Check sheet for the modelled part. Datum: model origin and axes. Units: mm. A direction names the side the tool comes from. Coordinates: 2 decimals unless noted, no trailing zeros. Write each loop counter-clockwise with the first axis right and the second up, starting at its lowest first coordinate (ties: lowest second). Pieces come first, ordered by that corner, then holes. Notation, with made-up numbers: (51, 30) - (87, 30) arc R14 cw to (87, 35) - close; hole circle Ø6 at (6.5, -7). An arc over 180 degrees is marked (long way). Answer as CSV lines item,"result". Start each with the question number.
from build123d import *

# Parameters (mm, degrees)
SKETCH_1_R      = 4
SKETCH_1_R_2    = 2.5
EXTRUDE_1_DEPTH = 6


with BuildPart() as part:
    # 스케치1 → 보스-돌출1 (new body)
    # profile 1 of 4: a face of its own
    with BuildSketch(Plane.XY):
        with BuildLine():
            Line((4, -3.202328983), (4, 0))
            ThreePointArc((4, 0), (-3e-09, -4), (-4, 6e-09))
            Line((-4, 6e-09), (-4, -1.928017797))
            Line((-4, -1.928017797), (-11.877068301, -1.928017797))
            Line((-11.877068301, -1.928017797), (-11.877068301, -4.928017797))
            Line((-11.877068301, -4.928017797), (-6.12956889, -4.928017797))
            Line((-6.12956889, -4.928017797), (-6.12956889, -7.005884989))
            Line((-6.12956889, -7.005884989), (1.618982626, -7.005884989))
            Line((1.618982626, -7.005884989), (4, -3.202328983))
        make_face()
    # profile 2 of 4: a face of its own
    with BuildSketch(Plane.XY):
        Circle(SKETCH_1_R)
        Circle(SKETCH_1_R_2, mode=Mode.SUBTRACT)
    # profile 3 of 4: a face of its own
    with BuildSketch(Plane.XY):
        with BuildLine():
            Line((4, 15), (-0.018657753, 12.499853249))
            Line((-0.018657753, 12.499853249), (-0.018657753, 8.804925293))
            Line((-0.018657753, 8.804925293), (-4, 6.585919306))
            Line((-4, 6.585919306), (-4, 6e-09))
            ThreePointArc((-4, 6e-09), (3e-09, 4), (4, 0))
            Line((4, 0), (4, 15))
        make_face()
    # profile 4 of 4: a face of its own
    with BuildSketch(Plane.XY):
        with BuildLine():
            ThreePointArc((-6.12956889, -7.005884989), (-9.072577994, -15.066190234), (-6.302707776, -23.187621278))
            ThreePointArc((-6.302707776, -23.187621278), (-4.499421911, -23.894054073), (-2.999999998, -22.668239597))
            ThreePointArc((-2.999999998, -22.668239597), (-3.892893232, -13.892647551), (1.618982626, -7.005884989))
            Line((1.618982626, -7.005884989), (-6.12956889, -7.005884989))
        make_face()
    extrude(amount=EXTRUDE_1_DEPTH)


solid = part.part
(1) Release check for a two-part mould opening along Y. For faces 4 (the face through (-3.928, -14.014, 2.958)), 5 (the face through (-6.13, -6, 3)), 6 (the face through (-4.53, -23.9, 2.96)), 7 (the face through (-0.019, 11, 3)) record: pulls with the +Y half, pulls with the -Y half, needs draft (parallel to the pull), parting line crosses it, or undercut.
(2) Cross-section at D-D on y = 12. Record the boundary of the cut face in (x, z).
(3) Go/stop test with flat-tipped pins: P1, Ø1.7, axis at x = -9, z = 4, coming from the -Y side; P2, Ø3, axis at y = 2.5, z = 3.5, coming from the -X side; P3, Ø3, axis at x = 0, y = 0, coming from the -Z side; P4, Ø0.6, axis at y = -6, z = 4.5, coming from the -X side. Record where each tip stops, or that it passes through.
(4) Material ranges on probe 1 along X at (y, z) = (-2, 2.95); probe 2 along X at (y, z) = (3.5, 4.25); probe 3 along X at (y, z) = (10.5, 3.8), recorded low to high. Write a range as from..to.
(5) Cross-section at A-A on y = 0. Record the boundary of the cut face in (x, z).
(6) Cross-section at B-B on z = 3.6. Record the boundary of the cut face in (x, y), plus the area to 3 significant figures.
(7) Tool access check on faces 1 (the face through (-9, -4.928, 3)), 2 (the face through (-11.877, -3, 3)), 3 (the face through (-4, 2, 3)). Record the directions out of +Z, -Z, +X, -X, +Y, -Y that give a thin tool (end or side, any length) a straight path to the whole face; none if there is none.
(8) Cross-section at C-C on x = -3.5. Record the boundary of the cut face in (y, z), plus the area to 3 significant figures.
Checked values:
1,face 4,"undercut"
1,face 5,"undercut"
1,face 6,"pulls with the -Y half"
1,face 7,"needs draft"
2,outline,"(-0.02, 0) - (4, 0) - (4, 6) - (-0.02, 6) - close"
3,P1,"y = -19.99"
3,P2,"x = -4"
3,P3,"through"
3,P4,"x = -6.13"
4,probe 1,"-11.88..-1.5, 1.5..4"
4,probe 2,"-4..4"
4,probe 3,"-0.02..4"
5,outline,"(-4, 0) - (-2.5, 0) - (-2.5, 6) - (-4, 6) - close; (2.5, 0) - (4, 0) - (4, 6) - (2.5, 6) - close"
6,outline,"(-11.88, -4.93) - (-6.13, -4.93) - (-6.13, -7.01) arc R12.89 ccw to (-6.3, -23.19) arc R1.92 ccw to (-3, -22.67) arc R11.65 cw to (1.62, -7.01) - (4, -3.2) - (4, 15) - (-0.02, 12.5) - (-0.02, 8.8) - (-4, 6.59) - (-4, -1.93) - (-11.88, -1.93) - close; hole circle Ø5 at (0, 0)"
6,area,"230 mm^2"
7,face 1,"+Z, -Z, -X"
7,face 2,"+Z, -Z, -X, +Y, -Y"
7,face 3,"+Z, -Z, -X, +Y"
8,outline,"(-23.41, 0) - (-21.6, 0) - (-21.6, 6) - (-23.41, 6) - close; (-12.77, 0) - (6.86, 0) - (6.86, 6) - (-12.77, 6) - close"
8,area,"129 mm^2"
